```python
from build123d import *

# Parameters (mm, degrees)
F0_W     = 114.3
F0_H     = 57.15
F1_DEPTH = 9.525
F2_R     = 5.08
F4_DEPTH = 9.525
F6_DEPTH = 9.525


with BuildPart() as f1:
    # F0 (on Top) → F1 (new body)
    with BuildSketch(Plane.XY):
        with Locations((-3.538748, -5.563198)):
            Rectangle(F0_W, F0_H)
    extrude(amount=F1_DEPTH)

    # F2
    f2_edges = [f1.edges().sort_by_distance(p)[0] for p in [
        (-60.688748, -34.138198, 4.7625),
        (53.611252, -34.138198, 4.7625),
    ]]
    fillet(f2_edges, radius=F2_R)

    # F3 (on Front) → F4 (join)
    with BuildSketch(Plane.XZ):
        with BuildLine():
            Line((41.378355, 0), (-48.737979, 0))
            Line((-48.737979, 0), (-48.737979, -25.4))
            ThreePointArc((-48.737979, -25.4), (-39.757723, -29.119744), (-36.037979, -38.1))
            Line((-36.037979, -38.1), (-16.379812, -38.1))
            ThreePointArc((-16.379812, -38.1), (-3.679812, -50.8), (9.020188, -38.1))
            Line((9.020188, -38.1), (28.678355, -38.1))
            ThreePointArc((28.678355, -38.1), (32.398099, -29.119744), (41.378355, -25.4))
            Line((41.378355, -25.4), (41.378355, 0))
        make_face()
    extrude(amount=F4_DEPTH)

    # F5 (on Right) → F6 (join)
    with BuildSketch(Plane.YZ):
        with BuildLine():
            Line((-9.288505, -38.1), (-9.288505, 0))
            Line((-9.288505, 0), (-29.608505, 0))
            Line((-29.608505, 0), (-29.608505, -1.29146))
            ThreePointArc((-29.608505, -1.29146), (-19.493946, -18.477158), (-15.944775, -38.1))
            Line((-15.944775, -38.1), (-9.288505, -38.1))
        make_face()
    extrude(amount=-F6_DEPTH)


solid = f1.part
```
Source: CAD feature listing. Evaluate the final solid. Frame: model axes, mm. A direction names the side the tool comes from. Give positions to 0.01 mm unless a question says otherwise; leave off trailing zeros. Order: outer loops, then holes, each group sorted by start corner. A loop starts at its lowest first (then second) coordinate and runs counter-clockwise, first axis right, second up.
(1) Section query D-D (y = 12.5). Return the cut outline in (x, z) (3 decimals), plus the area to 3 significant figures.
(2) Section query A-A (x = 26.5). Return the cut outline in (y, z) (3 decimals).
(3) Contact query for flat-ended pins moving along their axis: P1, Ø12, axis at x = -24.5, y = -3, coming from the -Z side; P2, Ø3, axis at x = -18.5, z = -38.5, coming from the +Y side; P3, Ø6, axis at y = -17, z = -12.5, coming from the -X side (3 decimals). Output: stop coordinate, or through.
(4) Access query for faces 4 (the face through (-14, -9.525, -19)), 5 (the face through (-9.525, -15, -15)), 6 (the face through (19, -5, -38.1)), 7 (the face through (-48.738, -5, -13)), 8 (the face through (-4, 0, -19)). Directions: +Z, -Z, +X, -X, +Y, -Y. A direction counts if a zero-diameter tool reaches every point of the face in a straight line with its end or side. Return the directions, or none.
(5) Material intervals for line 1 along Y through (x, z) = (32, -3) (3 decimals); line 2 along Z through (x, y) = (-47, 15) (3 decimals), sorted ascending.
(6) Section query B-B (y = -27.5). Return the cut outline in (x, z) (3 decimals), plus the area to 3 significant figures.
(7) Pull-direction query (Z, two-part tool) for faces 1 (the face through (-60.689, -3, 5)), 2 (the face through (-39.86, -4.7, -29.02)), 3 (the face through (-4, -5, 9.525)); classes: +Z half, -Z half, draft (parallel to the pull), parting line (faces both ways), or undercut.
(8) Section query C-C (y = -4). Return the cut outline in (x, z) (3 decimals), plus the area to 3 significant figures.
Outcome:
1. outline: (-60.689, 0) - (53.611, 0) - (53.611, 9.525) - (-60.689, 9.525) - close
1. area: 1,090 mm2
2. outline: (-34.138, 0) - (-9.525, 0) - (-9.525, -38.1) - (0, -38.1) - (0, 0) - (23.012, 0) - (23.012, 9.525) - (-34.138, 9.525) - close
3. P1: stops at z = -38.1
3. P2: stops at y = 0
3. P3: stops at x = -9.525
4. face 4: -Z, -Y
4. face 5: -Z, -X, -Y
4. face 6: -Z, +X, +Y, -Y
4. face 7: -Z, -X, +Y, -Y
4. face 8: -Z, +X, -X, +Y
5. line 1: y = -9.525 to 0
5. line 2: z = 0 to 9.525
6. outline: (-60.689, 0) - (-9.525, 0) - (-9.525, -3.905) - (0, -3.905) - (0, 0) - (53.611, 0) - (53.611, 9.525) - (-60.689, 9.525) - close
6. area: 1,130 mm2
7. face 1: draft
7. face 2: -Z half
7. face 3: +Z half
8. outline: (-60.689, 0) - (-48.738, 0) - (-48.738, -25.4) arc R12.7 cw to (-36.038, -38.1) - (-16.38, -38.1) arc R12.7 ccw to (9.02, -38.1) - (28.678, -38.1) arc R12.7 cw to (41.378, -25.4) - (41.378, 0) - (53.611, 0) - (53.611, 9.525) - (-60.689, 9.525) - close
8. area: 4,520 mm2
